from build123d import *

# Parameters (mm, degrees)
SKETCH_1_R      = 4
SKETCH_1_R_2    = 3
EXTRUDE_1_DEPTH = 90
EXTRUDE_START   = -90
SKETCH_2_R      = 3
EXTRUDE_2_DEPTH = 90


with BuildPart() as part:
    # 草图1 → 凸台-拉伸1 (new body)
    with BuildSketch(Plane.XY):
        with Locations(Location((0, 0, 0), (0, 0, 180))):
            Circle(SKETCH_1_R)
        with Locations(Location((0, 0, 0), (0, 0, 180))):
            Circle(SKETCH_1_R_2, mode=Mode.SUBTRACT)
    extrude(amount=EXTRUDE_1_DEPTH)

    # 草图2 → 凸台-拉伸2 (add)
    with BuildSketch(Plane.XY.offset(90).offset(EXTRUDE_START)):
        Polygon((4, 2.309401077), (0, 4.618802154), (-4, 2.309401077), (-4, -2.309401077), (0, -4.618802154), (4, -2.309401077), align=None)
        with Locations(Location((0, 0, 0), (0, 0, 180))):
            Circle(SKETCH_2_R, mode=Mode.SUBTRACT)
    extrude(amount=EXTRUDE_2_DEPTH)


solid = part.part
Verification items for the finished model (mm, model axes). Give positions to 0.01 mm unless a question says otherwise; leave off trailing zeros. Write each loop counter-clockwise with the first axis right and the second up, starting at its lowest first coordinate (ties: lowest second). Pieces come first, ordered by that corner, then holes. Notation, with made-up numbers: M 50.25,-39 L 91.25,-39 A33 cw 91.25,-6 Z; hole C 40,-18.75 d7. An arc over 180 degrees is marked long. Write item = value, one per line.
(1) Draft check along Y on faces 1 (the face through (-2.86, -0.9, 44.37)), 2 (the face through (-4, 0, 44)), 3 (the face through (1.97, -3.48, 44.37)). Enter one of: released by +Y, released by -Y, zero draft, split by the parting line, or undercut.
Found:
face_1 = undercut
face_2 = zero draft
face_3 = released by -Y
(2) Go/stop test with a flat-tipped pin: pin 1 Ø2 at (y, z) = (-2.5, 69) entering from -X. Record where the tip stops, or that it passes through.
Found:
pin_1 = -4
(3) Sectioned sample at B-B (z = 72). Record the cut outline in (x, y), then the cut area to 3 significant figures.
Found:
outline = M -4,-2.31 L 0,-4.62 L 4,-2.31 L 4,2.31 L 0,4.62 L -4,2.31 Z; hole C 0,0 d6
area = 27.2 mm2
(4) Sectioned sample at C-C (y = 0.75). Record the cut outline in (x, z), then the cut area to 3 significant figures.
Found:
outline = M -4,0 L -2.9,0 L -2.9,90 L -4,90 Z; M 2.9,0 L 4,0 L 4,90 L 2.9,90 Z
area = 197 mm2
(5) Material ranges on line 1 (Y direction, x = 0, z = 44); line 2 (Y direction, x = -2.75, z = 28); line 3 (X direction, y = 2.75, z = 72.5), recorded low to high.
Found:
line_1 = -4.62 to -3, 3 to 4.62
line_2 = -3.03 to -1.2, 1.2 to 3.03
line_3 = -3.24 to -1.2, 1.2 to 3.24
(6) Sectioned sample at A-A (x = -0.75). Record the cut outline in (y, z).
Found:
outline = M -4.19,0 L -2.9,0 L -2.9,90 L -4.19,90 Z; M 2.9,0 L 4.19,0 L 4.19,90 L 2.9,90 Z
